```python
from build123d import *

# Parameters (mm, degrees)
SKETCH_1_W          = 4
SKETCH_1_H          = 17
SKETCH_1_H_2        = 8
EXTRUDE_1_DEPTH     = 4
SKETCH_1_7_W        = 44.5
SKETCH_1_7_H        = 8
EXTRUDE_2_DEPTH     = 3.5
SKETCH_2_W          = 18.5
SKETCH_2_H          = 1.5
CUT_EXTRUDE_1_DEPTH = 34.705526253
SKETCH_2_3_W        = 2.5
SKETCH_2_3_H        = 1.5
EXTRUDE_4_DEPTH     = 25
FILLET_1_R          = 1
FILLET_2_R          = 1.5
FILLET_3_R          = 1
SKETCH_10_W         = 4.5
SKETCH_10_H         = 8
SKETCH_10_W_2       = 36
SKETCH_10_H_2       = 50
CUT_EXTRUDE_2_DEPTH = 45.331845213
CUT_EXTRUDE_3_DEPTH = 43.252958476
SKETCH_12_W         = 4
SKETCH_12_H         = 50
CUT_EXTRUDE_4_DEPTH = 2
SKETCH_13_R         = 0.6
CUT_EXTRUDE_5_DEPTH = 42.920311452
SKETCH_24_R         = 0.6
CUT_EXTRUDE_6_DEPTH = 42.920311452
SKETCH_25_W         = 9.588346595
SKETCH_25_H         = 3.3
CUT_EXTRUDE_7_DEPTH = 42.920311452
SKETCH_26_W         = 7.846978632
SKETCH_26_H         = 7.676354821
CUT_EXTRUDE_8_DEPTH = 39.99618586
SKETCH_27_W         = 71.858666529
SKETCH_27_H         = 35.216616035
CUT_EXTRUDE_9_DEPTH = 35.515395273


with BuildPart() as part:
    # 草图1 → 凸台-拉伸1 (new body)
    with BuildSketch(Plane(origin=(0, 0, 0), x_dir=(1, 0, 0), z_dir=(0, 1, 0))):
        with Locations((-15.75, -4)):
            Rectangle(SKETCH_1_W, SKETCH_1_H)
        with Locations((15.75, -4)):
            Rectangle(SKETCH_1_W, SKETCH_1_H)
        with Locations((15.75, 8.5)):
            Rectangle(SKETCH_1_W, SKETCH_1_H_2)
        with Locations((-15.75, 8.5)):
            Rectangle(SKETCH_1_W, SKETCH_1_H_2)
    extrude(amount=EXTRUDE_1_DEPTH)

    # 草图1<7> → 凸台-拉伸2 (add)
    with BuildSketch(Plane(origin=(0, 0, 0), x_dir=(1, 0, 0), z_dir=(0, 1, 0))):
        with Locations((0, 8.5)):
            Rectangle(SKETCH_1_7_W, SKETCH_1_7_H)
    extrude(amount=EXTRUDE_2_DEPTH)

    # 草图2 → 切除-拉伸1 (cut, through all)
    with BuildSketch(Plane(origin=(0, 0, -12.5), x_dir=(-1, 0, 0), z_dir=(0, 0, -1))):
        with Locations((0, 2.75)):
            Rectangle(SKETCH_2_W, SKETCH_2_H)
        Polygon((13.25, 3.5), (9.25, 3.5), (9.25, 2), align=None)
        Polygon((-9.25, 3.5), (-13.25, 3.5), (-9.25, 2), align=None)
        Polygon((-22.25, 3.5), (-22.25, 2), (-18.25, 3.5), align=None)
        Polygon((22.25, 3.5), (18.25, 3.5), (22.25, 2), align=None)
    extrude(amount=-CUT_EXTRUDE_1_DEPTH, mode=Mode.SUBTRACT)

    # 草图2<3> → 凸台-拉伸4 (add, through all)
    with BuildSketch(Plane(origin=(0, 0, -12.5), x_dir=(-1, 0, 0), z_dir=(0, 0, -1))):
        with Locations((-15.75, 7.25)):
            Rectangle(SKETCH_2_3_W, SKETCH_2_3_H)
        Polygon((-15, 6.5), (-16.5, 6.5), (-16.5, 4), (-15.75, 4), (-15, 4), align=None)
        with Locations((15.75, 7.25)):
            Rectangle(SKETCH_2_3_W, SKETCH_2_3_H)
        Polygon((16.5, 6.5), (15, 6.5), (15, 4), (15.75, 4), (16.5, 4), align=None)
    extrude(amount=-EXTRUDE_4_DEPTH)

    # 圆角1
    # the kernel refuses this fillet: 1 mm, written as the material it adds along each edge
    with BuildSketch(Plane(origin=(-16.5, 6.5, -12.5), x_dir=(-1, 0, 0), z_dir=(0, 0, 1)), Plane(origin=(15, 6.5, -12.5), x_dir=(-1, 0, 0), z_dir=(0, 0, 1))) as fillet_1_piece_1:
        with BuildLine():
            CenterArc((1, 0.866025404), FILLET_1_R, 180, 60)
            Line((0, 0.866025404), (-0.02, 0.866025404))
            Line((-0.02, 0.866025404), (-0.02, 0))
            Line((-0.02, 0), (0, -0.02))
            ThreePointArc((0, -0.02), (0.25, -0.02), (0.49, -0.017320508))
            Line((0.49, -0.017320508), (0.5, 0))
        make_face()
    extrude(amount=25)
    with BuildSketch(Plane(origin=(-15, 6.5, -12.5), x_dir=(0, -1, 0), z_dir=(0, 0, 1)), Plane(origin=(16.5, 6.5, -12.5), x_dir=(0, -1, 0), z_dir=(0, 0, 1))) as fillet_1_piece_2:
        with BuildLine():
            CenterArc((0.866025404, 1), FILLET_1_R, 210, 60)
            Line((0, 0.5), (-0.017320508, 0.49))
            ThreePointArc((-0.017320508, 0.49), (-0.02, 0.25), (-0.02, 0))
            Line((-0.02, 0), (0, -0.02))
            Line((0, -0.02), (0.866025404, -0.02))
            Line((0.866025404, -0.02), (0.866025404, 0))
        make_face()
    extrude(amount=25)

    # 圆角2
    # the kernel refuses this fillet: 1.5 mm, written as the material it adds along each edge
    with BuildSketch(Plane(origin=(16.5, 4, -12.5), x_dir=(1, 0, 0), z_dir=(0, 0, 1))) as fillet_2_piece_1:
        with BuildLine():
            CenterArc((1.5, 1.479019946), FILLET_2_R, 180, 80.405931773)
            Line((0, 1.479019946), (-0.03, 1.479019946))
            Line((-0.03, 1.479019946), (-0.03, 0))
            Line((-0.03, 0), (0, -0.03))
            ThreePointArc((0, -0.03), (0.625, -0.03), (1.245, -0.029580399))
            Line((1.245, -0.029580399), (1.25, 0))
        make_face()
    extrude(amount=25)
    with BuildSketch(Plane(origin=(15, 4, -12.5), x_dir=(0, 1, 0), z_dir=(0, 0, 1)), Plane(origin=(-16.5, 4, -12.5), x_dir=(0, 1, 0), z_dir=(0, 0, 1))) as fillet_2_piece_2:
        with BuildLine():
            CenterArc((1.479019946, 1.5), FILLET_2_R, 189.594068227, 80.405931773)
            Line((0, 1.25), (-0.029580399, 1.245))
            ThreePointArc((-0.029580399, 1.245), (-0.03, 0.625), (-0.03, 0))
            Line((-0.03, 0), (0, -0.03))
            Line((0, -0.03), (1.479019946, -0.03))
            Line((1.479019946, -0.03), (1.479019946, 0))
        make_face()
    extrude(amount=25)
    with BuildSketch(Plane(origin=(-15, 4, -12.5), x_dir=(0, 1, 0), z_dir=(0, 0, 1))) as fillet_2_piece_3:
        with BuildLine():
            CenterArc((1.479019946, -1.5), FILLET_2_R, 90, 80.405931773)
            Line((0, -1.25), (-0.029580399, -1.245))
            ThreePointArc((-0.029580399, -1.245), (-0.03, -0.625), (-0.03, 0))
            Line((-0.03, 0), (0, 0.03))
            Line((0, 0.03), (1.479019946, 0.03))
            Line((1.479019946, 0.03), (1.479019946, 0))
        make_face()
    extrude(amount=25)

    # 圆角3
    fillet_3_edges = [part.edges().sort_by_distance(p)[0] for p in [
        (14.5, 8, 0),
        (17, 8, 0),
        (-17, 8, 0),
        (-14.5, 8, 0),
    ]]
    fillet(fillet_3_edges, radius=FILLET_3_R)

    # 镜向2: part across plane


with BuildPart() as part_1:
    add(part.part)
    add(part.part.mirror(Plane(origin=(0, 4, 12.5), x_dir=(1, 0, 0), z_dir=(0, 0, -1))))

    # 草图10 → 切除-拉伸2 (cut, through all)
    with BuildSketch(Plane.XZ):
        with Locations((-20, 33.5)):
            Rectangle(SKETCH_10_W, SKETCH_10_H)
        with Locations((-20, -8.5)):
            Rectangle(SKETCH_10_W, SKETCH_10_H)
        with Locations((4.25, 12.5)):
            Rectangle(SKETCH_10_W_2, SKETCH_10_H_2)
    extrude(amount=-CUT_EXTRUDE_2_DEPTH, mode=Mode.SUBTRACT)

    # 草图11 → 切除-拉伸3 (cut, through all)
    with BuildSketch(Plane(origin=(0, 0, 0), x_dir=(-1, 0, 0), z_dir=(0, -1, 0))):
        with BuildLine():
            ThreePointArc((15.75, 12.5), (17.164213562, 11.914213562), (17.75, 10.5))
            Line((17.75, 10.5), (17.75, 12.5))
            Line((17.75, 12.5), (15.75, 12.5))
        make_face()
        with BuildLine():
            ThreePointArc((13.75, 10.5), (14.335786438, 11.914213562), (15.75, 12.5))
            Line((15.75, 12.5), (13.75, 12.5))
            Line((13.75, 12.5), (13.75, 10.5))
        make_face()
    extrude(amount=-CUT_EXTRUDE_3_DEPTH, mode=Mode.SUBTRACT)

    # 草图12 → 切除-拉伸4 (cut)
    with BuildSketch(Plane.XZ):
        with Locations((-15.75, 12.5)):
            Rectangle(SKETCH_12_W, SKETCH_12_H)
    extrude(amount=-CUT_EXTRUDE_4_DEPTH, mode=Mode.SUBTRACT)

    # 草图13 → 切除-拉伸5 (cut, through all)
    with BuildSketch(Plane(origin=(0, 8, 0), x_dir=(1, 0, 0), z_dir=(0, 1, 0))):
        with Locations(Location((-15.75, 10.5, 0), (0, 0, 270))):
            Circle(SKETCH_13_R)
    extrude(amount=-CUT_EXTRUDE_5_DEPTH, mode=Mode.SUBTRACT)

    # 草图16 → 切除-旋转1 (revolve, cut)
    with BuildSketch(Plane.XY.offset(37.5)):
        with BuildLine():
            Line((-17.75, 0), (-13.75, 0))
            Line((-13.75, 0), (-13.75, 4))
            ThreePointArc((-13.75, 4), (-14.645643924, 4.510774109), (-15, 5.479019946))
            Line((-15, 5.479019946), (-15, 5.633974596))
            ThreePointArc((-15, 5.633974596), (-14.866025404, 6.133974596), (-14.5, 6.5))
            Line((-14.5, 6.5), (-14.5, 7))
            ThreePointArc((-14.5, 7), (-14.792893219, 7.707106781), (-15.5, 8))
            Line((-15.5, 8), (-16, 8))
            ThreePointArc((-16, 8), (-16.707106781, 7.707106781), (-17, 7))
            Line((-17, 7), (-17, 6.5))
            ThreePointArc((-17, 6.5), (-16.633974596, 6.133974596), (-16.5, 5.633974596))
            Line((-16.5, 5.633974596), (-16.5, 5.479019946))
            ThreePointArc((-16.5, 5.479019946), (-16.854356076, 4.510774109), (-17.75, 4))
            Line((-17.75, 4), (-17.75, 0))
        make_face()
    revolve(axis=Axis((169.25, 37.729395322, 37.5), (0, -1, 0)), mode=Mode.SUBTRACT)

    # 草图24 → 切除-拉伸6 (cut, through all)
    with BuildSketch(Plane(origin=(0, 2, 0), x_dir=(-1, 0, 0), z_dir=(0, -1, 0))):
        with Locations(Location((15.75, 5.5, 0), (0, 0, 90))):
            Circle(SKETCH_24_R)
    extrude(amount=-CUT_EXTRUDE_6_DEPTH, mode=Mode.SUBTRACT)

    # 草图25 → 切除-拉伸7 (cut, through all)
    with BuildSketch(Plane(origin=(0, 8, 0), x_dir=(1, 0, 0), z_dir=(0, 1, 0))):
        with Locations((-13.334902889, -35.85)):
            Rectangle(SKETCH_25_W, SKETCH_25_H)
    extrude(amount=-CUT_EXTRUDE_7_DEPTH, mode=Mode.SUBTRACT)

    # 草图26 → 切除-拉伸8 (cut, through all)
    with BuildSketch(Plane(origin=(0, 8, 0), x_dir=(1, 0, 0), z_dir=(0, 1, 0))):
        with Locations((-16.033810668, -32.338177411)):
            Rectangle(SKETCH_26_W, SKETCH_26_H)
    extrude(amount=-CUT_EXTRUDE_8_DEPTH, mode=Mode.SUBTRACT)


with BuildPart() as body_2:
    # 镜向3: mirrored copy
    add(part_1.part.mirror(Plane(origin=(0, 0, 0), x_dir=(0, 0, 1), z_dir=(1, 0, 0))))


with BuildPart() as part_2:
    add(part_1.part)

    # 草图27 → 切除-拉伸9 (cut, through all)
    with BuildSketch(Plane(origin=(0, 0, 0), x_dir=(0, 0, -1), z_dir=(1, 0, 0))):
        with Locations((-17.475525281, 10.465734061)):
            Rectangle(SKETCH_27_W, SKETCH_27_H)
    extrude(amount=-CUT_EXTRUDE_9_DEPTH, mode=Mode.SUBTRACT)


solid = body_2.part
```
Geometry: final body of the model. Coordinates: model frame, mm. A direction names the side the tool comes from. Coordinates: 2 decimals unless noted, no trailing zeros. Order: outer loops, then holes, each group sorted by start corner. A loop starts at its lowest first (then second) coordinate and runs counter-clockwise, first axis right, second up. Notation, with made-up numbers: M 65.5,71 L 91.5,71 A32 ccw 91.5,110 Z; hole C 25.25,-17 d3. An arc over 180 degrees is marked long. Answer in a Markdown table with one row per item. Add a question column.
Q1. Section query B-B on z = -5.5. Return the cut outline in (x, y), and give its area (3 significant figures).
Q2. Reachability of faces 1 (the cylindrical face through (14.862, 6.14, 0.978)), 2 (the cylindrical face through (16.254, 2.986, 13.896)), 3 (the cylindrical face through (16.864, 4.5, 8.359)) from +Z, -Z, +X, -X, +Y, -Y: full face, straight path, thin tool, end or side. Return the list, or none.
Q3. Line query: L1, parallel to X at y = 3.5, z = -5.5; L2, parallel to X at y = 5.5, z = 2; L3, parallel to Y at x = 16.75, z = 24. Output: solid intervals per line, ascending.
Q4. Section query A-A on y = 3.5. Return the cut outline in (x, z).
Q5. Contact query for flat-ended pins moving along their axis: P1, Ø1.5, axis at y = 6, z = 17.5, coming from the -X side; P2, Ø2, axis at y = 7, z = -2, coming from the +X side; P3, Ø1.5, axis at y = 4.5, z = 16, coming from the -X side. Output: stop coordinate, or through.
Q6. Section query C-C on y = 5. Return the cut outline in (x, z).
Q7. Mould query, pull axis X, two halves, no side actions, for faces 4 (the flat face through (13.75, 3, -6)), 5 (the flat face through (17.75, 3, 9)), 6 (the cylindrical face through (15.34, 5.04, -10.94)). Classes: released by +X, released by -X, zero draft, split by the parting line, or undercut.
Completed:
| question | item | result |
|---|---|---|
| 1 | outline | M 13.75,2 L 15.15,2 L 15.15,7.94 A1 ccw 14.5,7 L 14.5,6.5 A1 cw 15,5.63 L 15,5.48 A1.5 cw 13.75,4 Z; M 16.35,2 L 17.75,2 L 17.75,4 A1.5 cw 16.5,5.48 L 16.5,5.63 A1 cw 17,6.5 L 17,7 A1 ccw 16.35,7.94 Z |
| 1 | area | 9.05 mm2 |
| 2 | face 1 | +Z, -Z, -X |
| 2 | face 2 | +Z, -X, -Y |
| 2 | face 3 | +Z, -Z, +X |
| 3 | L1 | x = 13.75 to 15.15, 16.35 to 17.75 |
| 3 | L2 | x = 15 to 16.5 |
| 3 | L3 | y = 4.19 to 4.65, 6.3 to 7.66 |
| 4 | outline | M 13.75,-10.5 A2 ccw 17.75,-10.5 L 17.75,28.5 L 17.53,28.5 A187 cw 13.75,-0.97 Z; hole C 15.75,-10.5 d1.2; hole C 15.75,-5.5 d1.2 |
| 5 | P1 | stops at x = 15.35 |
| 5 | P2 | stops at x = 17 |
| 5 | P3 | stops at x = 15.24 |
| 6 | outline | M 14.92,-12.32 A2 ccw 16.58,-12.32 L 16.58,28.5 L 16.36,28.5 A185.83 cw 14.92,12.74 Z; hole C 15.75,-10.5 d1.2; hole C 15.75,-5.5 d1.2 |
| 7 | face 4 | released by -X |
| 7 | face 5 | released by +X |
| 7 | face 6 | undercut |
